Answer from the drawing. Dimensions are ordinates in mm from the lowest x, y and z of the part. A direction names the side the tool comes from. Give positions to 0.01 mm unless a question says otherwise; leave off trailing zeros. Write each loop counter-clockwise with the first axis right and the second up, starting at its lowest first coordinate (ties: lowest second). Pieces come first, ordered by that corner, then holes.
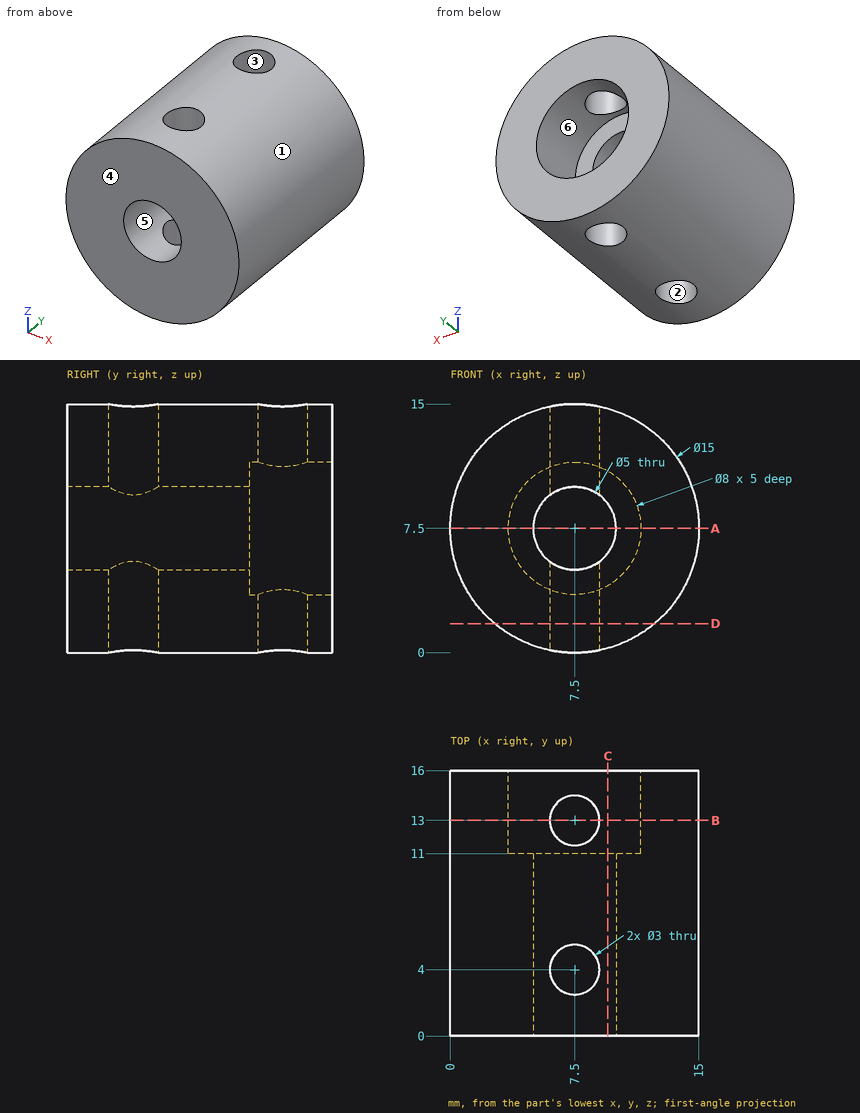
Item 1: A cutting plane is placed at D-D, the plane z = 1.75. Give the vertices of the cut face in (x, y).
Conclusion:
outline: (2.68, 0) - (12.32, 0) - (12.32, 16) - (2.68, 16) - close; hole circle Ø3 at (7.5, 4); hole circle Ø3 at (7.5, 13)
Item 2: Determine the mould class of the marked faces 1, 2, 3 and 4 for opening direction X: pulls with the +X half, pulls with the -X half, needs draft (parallel to the pull), parting line crosses it, or undercut.
Conclusion:
face 1: parting line crosses it
face 2: undercut
face 3: undercut
face 4: needs draft
Item 3: Which of the six approach directions +Z, -Z, +X, -X, +Y, -Y give full straight-line access (tool end or side, diameter ignored) to the marked faces 5 and 6?
Conclusion:
face 5: +Y, -Y
face 6: +Y
Item 4: Each of these flat-tipped pins is pushed along its axis until it touches: P1, Ø2, axis at y = 6, z = 5, coming from the -X side; P2, Ø1.8, axis at x = 7.5, y = 13, coming from the +Z side; P3, Ø6, axis at x = 3.5, y = 9.5, coming from the +Z side; P4, Ø6, axis at y = 11, z = 13, coming from the -X side. Where does it stop, or does it pass through?
Conclusion:
P1: stops at x = 0.15
P2: passes through
P3: stops at z = 14.93
P4: stops at x = 0.43
Item 5: A cutting plane is placed at B-B, the plane y = 13. Give the vertices of the cut face in (x, z).
Conclusion:
outline: (6, 0.15) - (6, 3.79) arc R4 cw to (6, 11.21) - (6, 14.85) arc R7.5 ccw to start; (9, 0.15) arc R7.5 ccw to (9, 14.85) - (9, 11.21) arc R4 cw to (9, 3.79) - close
Item 6: Consider probe 1 along X at (y, z) = (7.25, 7.5); probe 2 along X at (y, z) = (10.25, 6.5); probe 3 along Y at (x, z) = (8.5, 3). Determine where each line is inside the solid, lowest interval first.
Conclusion:
probe 1: x = 0 to 5, 10 to 15
probe 2: x = 0.07 to 5.21, 9.79 to 14.93
probe 3: y = 0 to 2.88, 5.12 to 11.88, 14.12 to 16
Item 7: A cutting plane is placed at A-A, the plane z = 7.5. Give the vertices of the cut face in (x, y).
Conclusion:
outline: (0, 0) - (5, 0) - (5, 11) - (3.5, 11) - (3.5, 16) - (0, 16) - close; (10, 0) - (15, 0) - (15, 16) - (11.5, 16) - (11.5, 11) - (10, 11) - close
Item 8: A cutting plane is placed at C-C, the plane x = 9.5. Give the vertices of the cut face in (y, z), plus the area to 3 significant figures.
Conclusion:
outline: (0, 0.27) - (16, 0.27) - (16, 4.04) - (11, 4.04) - (11, 6) - (0, 6) - close; (0, 9) - (11, 9) - (11, 10.96) - (16, 10.96) - (16, 14.73) - (0, 14.73) - close
area: 164 mm2
